Autodesk Inventor part; units mm, degrees
ref_plane "YZ Plane" through (0, 0, 0) normal (1, 0, 0) x (0, 1, 0)
ref_plane "XZ Plane" through (0, 0, 0) normal (0, 1, 0) x (-1, 0, 0)
ref_plane "XY Plane" through (0, 0, 0) normal (0, 0, 1) x (1, 0, 0)
sketch "Skizze1" plane through (0, 0, 0) normal (0, 0, 1) x (1, 0, 0)
  line L0 (17.8939, 18.6723) -> (2.8939, 18.6723)
  line L1 (2.8939, 18.6723) -> (2.8939, 15.6723)
  line L2 (2.8939, 15.6723) -> (17.8939, 15.6723)
  line L3 (17.8939, 15.6723) -> (17.8939, 18.6723)
  line L4 (17.8939, 9.0723) -> (2.8939, 9.0723)
  line L5 (2.8939, 9.0723) -> (2.8939, 6.0723)
  line L6 (2.8939, 6.0723) -> (17.8939, 6.0723)
  line L7 (17.8939, 6.0723) -> (17.8939, 9.0723)
  line L8 (17.8939, 15.6723) -> (17.8939, 12.3723) construction
  line L9 (17.8939, 12.3723) -> (17.8939, 9.0723) construction
  point P0 (0, 0)
  point P1 (10.3939, 9.0723)
  dimension "d0" = 15
  dimension "d1" = 3
  dimension "d2" = 3
  dimension "d3" = 6.6
extrude "Extrusion1" add sketch "Skizze1" along normal blind 21
chamfer "Fasen1" distance 5 distance2 21 1 edges at (17.8939, 7.5723, 21) measured on face at (7.8939, 8.0723, 21)
chamfer "Fasen2" distance 5 distance2 21 1 edges at (17.8939, 17.1723, 21) measured on face at (7.8939, 17.6723, 21)
fillet "Rundung1" radius 3 4 edges at (2.8939, 17.1723, 21) (2.8939, 7.5723, 21) (12.8944, 17.1723, 21) (12.8944, 7.5723, 21)
sketch "Skizze2" plane through (2.8939, 6.0723, 0) normal (0, -1, 0) x (1, 0, 0)
  circle A0 centre (5.587, 15.413) radius 5.587 construction
  line L0 (0, 0) -> (0, 21) construction
  line L1 (5.587, 15.413) -> (5.587, 21)
  line L2 (5.587, 15.413) -> (0, 15.413)
  line L3 (3, 21) -> (7.6304, 21)
  line L4 (10.5488, 18.6949) -> (15, 0)
  point P0 (-2.8939, 0)
  point P1 (0, 18)
hole "Bohrung1" at (8.4809, 6.0723, 15.413) direction (0, 1, 0) diameter 3.242 end through all countersink diameter 9 countersink angle 90
sketch "Skizze3" plane through (2.8939, 15.6723, 0) normal (0, -1, 0) x (1, 0, 0)
  line L0 (0, 0) -> (15, 0)
  line L1 (15, 0) -> (14.0476, 4)
  line L2 (14.0476, 4) -> (0, 4)
  line L3 (0, 0) -> (0, 21)
  line L4 (15, 0) -> (10.5488, 18.6949)
  point P0 (-2.8939, 0)
  point P1 (0, 18)
  dimension "d51" = 4
extrude "Extrusion2" add sketch "Skizze3" along normal through all
sketch "Skizze4" plane through (2.8939, 15.6723, 4) normal (0, 0, 1) x (1, 0, 0)
  line L0 (7.6304, 3) -> (3, 3) construction
  line L1 (3, -3.3) -> (11, -3.3)
  line L2 (3, -3.3) -> (0, -3.3)
  line L3 (0, 0) -> (0, -6.6)
  line L4 (14.0476, 0) -> (14.0476, -6.6)
  point P0 (12, 3)
  point P1 (14.0476, -3.3)
  point P2 (14.5, 0)
  dimension "d48" = 8
  dimension "d49" = 3
  dimension "d50" = 3.0476
hole "Bohrung2" at (13.8939, 12.3723, 4) at (5.8939, 12.3723, 4) direction (0, 0, -1) diameter 3.2 end through all countersink diameter 6.3 countersink angle 90
sketch "Skizze5" plane through (2.8939, 6.0723, 0) normal (0, -1, 0) x (1, 0, 0)
  circle A0 centre (5.587, 15.413) radius 4.5
  point P0 (-2.8939, 0)
  point P1 (11.255, 14.9799)
  point P2 (11.9803, 12.079)
hole "Bohrung3" at (8.4809, 6.0723, 15.413) direction (0, 1, 0) diameter 4.3 depth 3
properties part number "HalterUmlenkrolleH" material "Aluminium 6061(1)"
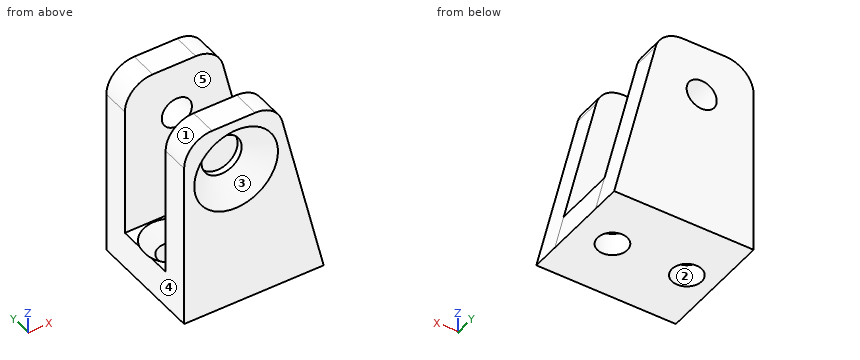
Source: CAD feature listing. Evaluate the final solid. Frame: model axes, mm. Face numbers are marked on the shaded views. A direction names the side the tool comes from. Give positions to 0.01 mm unless a question says otherwise; leave off trailing zeros. Order: outer loops, then holes, each group sorted by start corner. A loop starts at its lowest first (then second) coordinate and runs counter-clockwise, first axis right, second up.
(1) Section query A-A (z = 5.25). Return the cut outline in (x, y), plus the area to 3 significant figures.
(2) Access query for the marked faces 4 and 5. Directions: +Z, -Z, +X, -X, +Y, -Y. A direction counts if a zero-diameter tool reaches every point of the face in a straight line with its end or side. Return the directions, or none.
(3) Contact query for flat-ended pins moving along their axis: P1, Ø5, axis at x = 13.89, y = 12.37, coming from the +Z side; P2, Ø4.5, axis at x = 10.5, z = 14.5, coming from the -Y side; P3, Ø5, axis at x = 8.48, z = 15.41, coming from the -Y side. Output: stop coordinate, or through.
(4) Section query C-C (y = 12.75). State how many separate pieces and enclosed holes the cut face has, plus the area to 3 significant figures.
(5) Material intervals for line 1 along Y through (x, z) = (7.25, 8); line 2 along Z through (x, y) = (8.5, 9); line 3 along Z through (x, y) = (6.75, 7.75), sorted ascending.
(6) Pull-direction query (Y, two-part tool) for the marked faces 1, 2 and 3; classes: +Y half, -Y half, draft (parallel to the pull), parting line (faces both ways), or undercut.
Outcome:
1. outline: (2.89, 6.07) - (16.64, 6.07) - (16.64, 9.07) - (2.89, 9.07) - close; (2.89, 15.67) - (16.64, 15.67) - (16.64, 18.67) - (2.89, 18.67) - close
1. area: 82.5 mm2
2. face 4: +Z, -Z, -X, +Y, -Y
2. face 5: +Z, +X, -X
3. P1: stops at z = 3.35
3. P2: stops at y = 6.11
3. P3: stops at y = 8.07
4. separate pieces: 3
4. enclosed holes: 0
4. area: 28.3 mm2
5. line 1: y = 6.07 to 9.07, 15.67 to 18.67
5. line 2: z = 0 to 13.26, 17.56 to 21
5. line 3: z = 0 to 13.18, 17.64 to 21
6. face 1: draft
6. face 2: undercut
6. face 3: -Y half
